Input: dimensioned drawing with shaded views. Units: mm. Origin: part minimum x, y, z. A direction names the side the tool comes from. Round coordinates to 2 decimals unless told otherwise and drop trailing zeros. Answer as a JSON object with one key per item and string values. Group by question number.
Item 1: Draft query along X for the marked faces 3 and 4. Return one class per face: released by +X, released by -X, zero draft, split by the parting line, or undercut.
Item 2: Line query: line 1 (X direction, y = 14.25, z = 2) (1 decimal); line 2 (Y direction, x = 12.75, z = 7.25); line 3 (Y direction, x = 11.5, z = 5) (1 decimal). Output: solid intervals per line, ascending.
Item 3: First-contact query: pin 1 (1 mm diameter, centred on y = 8, z = 8, fed in from +X) (1 decimal); pin 2 (3 mm diameter, centred on y = 19.5, z = 6, fed in from +X); pin 3 (5 mm diameter, centred on y = 4.5, z = 5, fed in from +X). Flat tips, straight axial feed; report the tip coordinate or a pass-through.
Item 4: Reachability of the marked faces 1 and 2 from +Z, -Z, +X, -X, +Y, -Y: full face, straight path, thin tool, end or side. Return the list, or none.
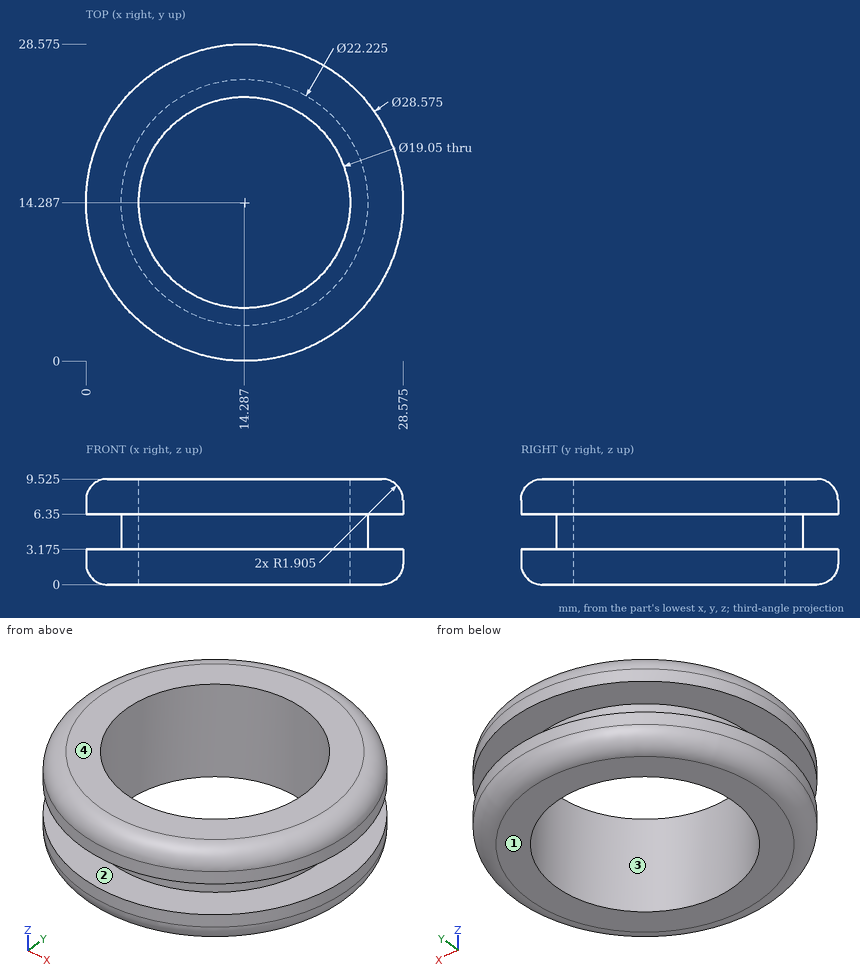
Values:
{
 "1": {"face 3": "undercut", "face 4": "zero draft"},
 "2": {"line 1": "x = 0 to 4.8, 23.8 to 28.6", "line 2": "y = 0.08 to 4.89, 23.69 to 28.49", "line 3": "y = 3.5 to 5.2, 23.4 to 25"},
 "3": {"pin 1": "stops at x = 27.3", "pin 2": "stops at x = 28.07", "pin 3": "stops at x = 26.33"},
 "4": {"face 1": "-Z, +X, -X, +Y, -Y", "face 2": "none"}
}
